Source: three-view drawing plus pictorial views. Frame: mm from the lowest corner of the part. A direction names the side the tool comes from. Round coordinates to 2 decimals unless told otherwise and drop trailing zeros. Loops run counter-clockwise (first coordinate to the right, second up) from the corner with the lowest first, then second, coordinate; pieces in that order, holes last. Notation, with made-up numbers: (59, -27) -> (72, -27) arc R31 ccw to (72, 9) -> close; hole circle Ø9 at (40.5, 16). An arc over 180 degrees is marked (long way). Answer as a JSON object with one key per item and string values. Group by question number.
Item 1: Section query B-B on x = 1.6. Return loops of the section in (y, z).
Item 2: Pin query (flat end, axial travel): pin 1 (1 mm diameter, centred on x = 3.5, y = 9, fed in from +Z). Return the tip coordinate at first contact, or that it passes through.
Item 3: Set-up query: the marked faces 1 and 2. Return all of +Z, -Z, +X, -X, +Y, -Y with unobstructed straight access to the full face (end or side cutting, diameter ignored); none if empty.
Item 4: Draft query along Z for the marked faces 3, 4 and 5. Return one class per face: released by +Z, released by -Z, zero draft, split by the parting line, or undercut.
Item 5: Section query C-C on z = 2.05. Return loops of the section in (x, y).
Item 6: Section query D-D on y = 17.25. Return loops of the section in (x, z) (1 decimal).
Item 7: Material intervals for line 1 (Y direction, x = 2.15, z = 1.95); line 2 (Y direction, x = 0.4, z = 1.5); line 3 (X direction, y = 2, z = 3.1) (1 decimal), sorted ascending. Write a range as [from, to].
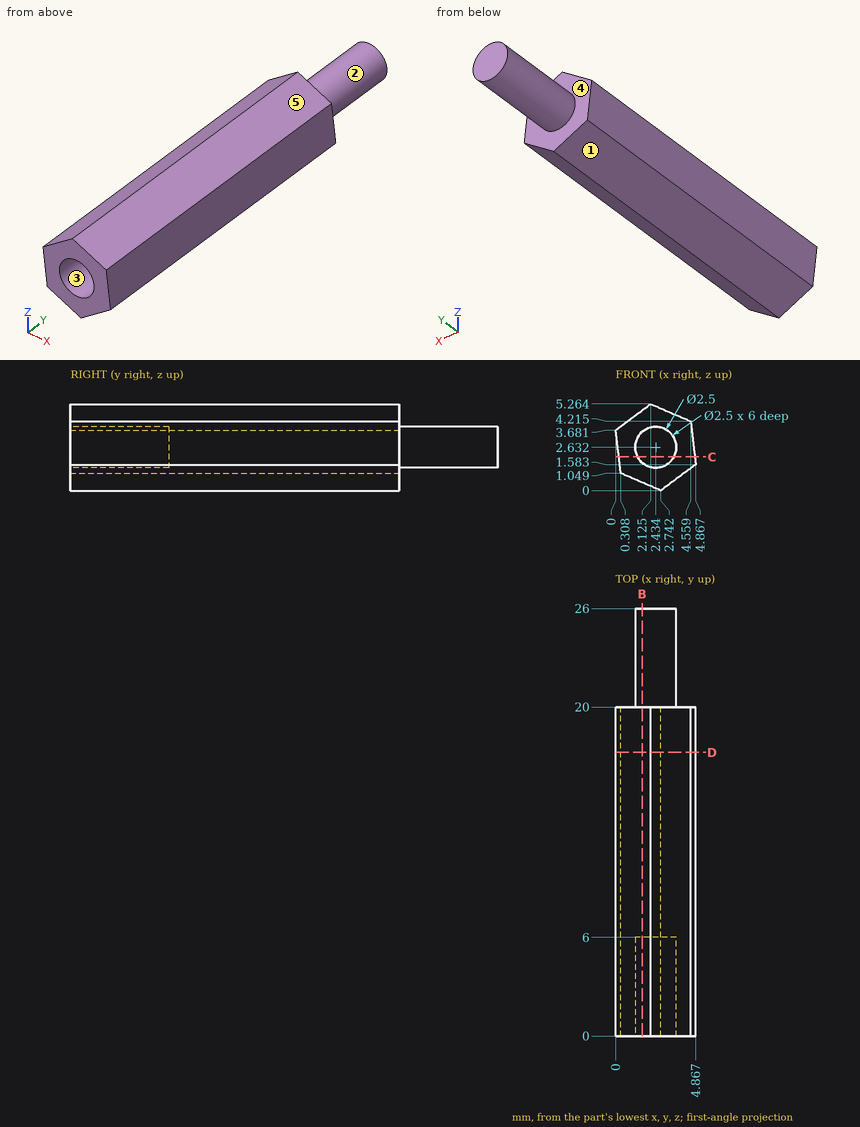
Solved:
{
 "1": {"outline": "(0, 0.49) -> (20, 0.49) -> (20, 1.7) -> (26, 1.7) -> (26, 3.56) -> (20, 3.56) -> (20, 4.87) -> (0, 4.87) -> (0, 3.56) -> (6, 3.56) -> (6, 1.7) -> (0, 1.7) -> close"},
 "2": {"pin 1": "z = 4.89"},
 "3": {"face 1": "-Z, -X, +Y, -Y", "face 2": "+Y"},
 "4": {"face 3": "undercut", "face 4": "zero draft", "face 5": "released by +Z"},
 "5": {"outline": "(0.19, 0) -> (1.33, 0) -> (1.33, 6) -> (3.54, 6) -> (3.54, 0) -> (4.81, 0) -> (4.81, 20) -> (3.54, 20) -> (3.54, 26) -> (1.33, 26) -> (1.33, 20) -> (0.19, 20) -> close"},
 "6": {"outline": "(0, 3.7) -> (0.3, 1) -> (2.7, 0) -> (4.9, 1.6) -> (4.6, 4.2) -> (2.1, 5.3) -> close"},
 "7": {"line 1": "[6, 26]", "line 2": "[0, 20]", "line 3": "[0.1, 1.3], [3.6, 4.7]"}
}
